from build123d import *

# Parameters (mm, degrees)
SKETCH1_R                = 1.1
SKETCH1_W                = 10
SKETCH1_H                = 2.49
BOSS_EXTRUDE1_DEPTH      = 1.67
SKETCH2_W                = 9.5
SKETCH2_H                = 9.5
BOSS_EXTRUDE2_DEPTH      = 5
SKETCH3_R                = 3.75
BOSS_EXTRUDE3_DEPTH      = 1
FILLET1_R                = 1
SKETCH4_W                = 9.5
SKETCH4_H                = 4.61
BOSS_EXTRUDE4_DEPTH      = 1
SKETCH5_W                = 8.8
SKETCH5_H                = 3.91
BOSS_EXTRUDE5_DEPTH      = 2
CHAMFER1_SIZE            = 0.65
BOSS_EXTRUDE6_DEPTH      = 2.75
BOSS_EXTRUDE6_DEPTH_BACK = 2.75
SKETCH7_W                = 22
SKETCH7_H                = 1
BOSS_EXTRUDE7_DEPTH      = 2.6
SKETCH9_W                = 21.8
SKETCH9_H                = 4
BOSS_EXTRUDE8_DEPTH      = 2.5


with BuildPart() as part:
    # Sketch1 → Boss-Extrude1 (new body)
    with BuildSketch(Plane.XY):
        with BuildLine():
            Line((-10.5, -11.93), (10.5, -11.93))
            ThreePointArc((10.5, -11.93), (11.914213562, -11.344213562), (12.5, -9.93))
            Line((12.5, -9.93), (12.5, 9.93))
            ThreePointArc((12.5, 9.93), (11.914213562, 11.344213562), (10.5, 11.93))
            Line((10.5, 11.93), (-10.5, 11.93))
            ThreePointArc((-10.5, 11.93), (-11.914213562, 11.344213562), (-12.5, 9.93))
            Line((-12.5, 9.93), (-12.5, -9.93))
            ThreePointArc((-12.5, -9.93), (-11.914213562, -11.344213562), (-10.5, -11.93))
        make_face()
        with Locations((-10.5, 9.93)):
            Circle(SKETCH1_R, mode=Mode.SUBTRACT)
        with Locations((10.5, 9.93)):
            Circle(SKETCH1_R, mode=Mode.SUBTRACT)
        with Locations((-10.5, -2.57)):
            Circle(SKETCH1_R, mode=Mode.SUBTRACT)
        with Locations((10.5, -2.57)):
            Circle(SKETCH1_R, mode=Mode.SUBTRACT)
        with Locations((0, 4.965)):
            Rectangle(SKETCH1_W, SKETCH1_H, mode=Mode.SUBTRACT)
    extrude(amount=BOSS_EXTRUDE1_DEPTH)

    # Sketch2 → Boss-Extrude2 (add)
    with BuildSketch(Plane.XY.offset(1.67)):
        with Locations((0, -2.57)):
            Rectangle(SKETCH2_W, SKETCH2_H)
    extrude(amount=BOSS_EXTRUDE2_DEPTH)

    # Sketch3 → Boss-Extrude3 (add)
    with BuildSketch(Plane.XY.offset(6.67)):
        with Locations((0, -2.57)):
            Circle(SKETCH3_R)
    extrude(amount=BOSS_EXTRUDE3_DEPTH)

    # Fillet1
    fillet1_edges = [part.edges().sort_by_distance(p)[0] for p in [
        (-3.75, -2.57, 7.67),
    ]]
    fillet(fillet1_edges, radius=FILLET1_R - 0.0001)  # a hair under: the kernel refuses the full size

    # Sketch4 → Boss-Extrude4 (add)
    with BuildSketch(Plane.XY.offset(1.67)):
        with Locations((0, -9.625)):
            Rectangle(SKETCH4_W, SKETCH4_H)
    extrude(amount=BOSS_EXTRUDE4_DEPTH)

    # Sketch5 → Boss-Extrude5 (add)
    with BuildSketch(Plane.XY.offset(2.67)):
        with Locations((0, -9.625)):
            Rectangle(SKETCH5_W, SKETCH5_H)
    extrude(amount=BOSS_EXTRUDE5_DEPTH)

    # Chamfer1
    chamfer1_edges = [part.edges().sort_by_distance(p)[0] for p in [
        (4.4, -9.625, 4.67),
        (0, -7.67, 4.67),
        (-4.4, -9.625, 4.67),
        (0, -11.58, 4.67),
    ]]
    chamfer(chamfer1_edges, length=CHAMFER1_SIZE)

    # Sketch6 → Boss-Extrude6 (add, two sides: drawn at the far end of the back side and taken through both)
    with BuildSketch(Plane(origin=(0, 0, 0), x_dir=(0, 0, -1), z_dir=(1, 0, 0)).offset(-BOSS_EXTRUDE6_DEPTH_BACK)):
        with BuildLine():
            Line((-3.298312235, 2.18), (-3.534834551, 2.18))
            add(Edge.make_bspline(
                [(-3.534834551, 2.18), (-3.534834551, 4.944931667), (-0.47055609, 4.534187875), (0.730328755, 6.849182289), (0.79246314, 7.291776262), (0.79246314, 7.33)],
                knots=[0, 0, 0, 0, 0.784106591, 0.986086671, 1, 1, 1, 1], degree=3))
            Line((0.79246314, 7.33), (0, 7.33))
            Line((0, 7.33), (0, 11.83))
            Line((0, 11.83), (1.2, 11.83))
            Line((1.2, 11.83), (1.2, 7.33))
            Line((1.2, 7.33), (1.028985456, 7.33))
            add(Edge.make_bspline(
                [(-3.298312235, 2.18), (-3.298312235, 2.369708531), (-3.268931161, 2.774833109), (-3.111748266, 3.367193807), (-2.767956088, 3.909628415), (-2.161529025, 4.362480865), (-1.410396471, 4.725696596), (-0.605704822, 5.099255509), (0.165819225, 5.601384629), (0.682287807, 6.265090703), (0.910091228, 6.771630764), (0.98633259, 7.041505733), (1.014862156, 7.172550739), (1.028985456, 7.28085491), (1.028985456, 7.33)],
                knots=[0, 0, 0, 0, 0.0625, 0.125, 0.25, 0.375, 0.5, 0.625, 0.75, 0.875, 0.9375, 0.96875, 0.984375, 1, 1, 1, 1], degree=3))
        make_face()
    extrude(amount=BOSS_EXTRUDE6_DEPTH + BOSS_EXTRUDE6_DEPTH_BACK)

    # Sketch7 → Boss-Extrude7 (add)
    with BuildSketch(Plane(origin=(0, 0, 0), x_dir=(-1, 0, 0), z_dir=(0, 0, -1))):
        with Locations((0, -11.33)):
            Rectangle(SKETCH7_W, SKETCH7_H)
    extrude(amount=BOSS_EXTRUDE7_DEPTH)

    # Sketch9 → Boss-Extrude8 (add)
    with BuildSketch(Plane(origin=(0, 0, 0), x_dir=(-1, 0, 0), z_dir=(0, 0, -1))):
        with Locations((0, -8.83)):
            Rectangle(SKETCH9_W, SKETCH9_H)
    extrude(amount=BOSS_EXTRUDE8_DEPTH)


solid = part.part
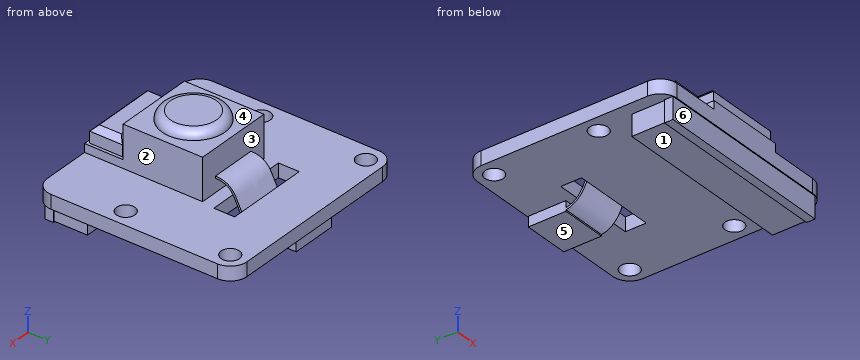
Build history of the part. All positions in model axes, mm. Face numbers are marked on the shaded views. A direction names the side the tool comes from. Coordinates: 2 decimals unless noted, no trailing zeros. Write each loop counter-clockwise with the first axis right and the second up, starting at its lowest first coordinate (ties: lowest second). Pieces come first, ordered by that corner, then holes.
(1) 3-axis set-ups, long thin cutter, end or side, ignore diameter. For the marked faces 4, 5 and 6: which of +Z, -Z, +X, -X, +Y, -Y reach the whole face in a straight line?
(2) Cut at B-B on y = -2.57. State how many separate pieces and enclosed holes the cut face has, and give its area (3 significant figures).
(3) Pin check, flat tips, straight feed: pin 1 Ø1.2 at (y, z) = (-8, -1.5) entering from -X; pin 2 Ø1.5 at (x, z) = (0, 3) entering from +Y; pin 3 Ø1.3 at (x, y) = (-1.5, -9.5) entering from +Z; pin 4 Ø1 at (x, z) = (5.5, 5) entering from +Y. Stop position of each tip, or through.
(4) Cut at A-A on x = 8.75. List the corners of the cut face in (y, z).
(5) Cut at D-D on z = 6.25. List the corners of the cut face in (x, y), and give its area (4 significant figures).
(6) Mould opens along Z. For the marked faces 1, 2 and 3 say: pulls with the +Z half, pulls with the -Z half, needs draft (parallel to the pull), parting line crosses it, or undercut.
(7) Drill centre lines: line 1 (Y direction, x = 10.5, z = 1.05); line 2 (Y direction, x = -1.25, z = 0.5); line 3 (Z direction, x = 1.75, y = 2.25). Where is each one in solid material? Low to high.
(8) Cut at C-C on z = -1.75. List the corners of the cut face in (x, y), and give its area (3 significant figures).
Working result:
1. face 4: +Z
1. face 5: -Z, +X, -X, +Y
1. face 6: -Z, +X, -X, -Y
2. separate pieces: 3
2. enclosed holes: 0
2. area: 89.0 mm2
3. pin 1: stops at x = -10.9
3. pin 2: stops at y = 4.56
3. pin 3: stops at z = 4.67
3. pin 4: passes through
4. outline: (-11.93, 0) - (-11.83, 0) - (-11.83, -2.6) - (-10.83, -2.6) - (-10.83, -2.5) - (-6.83, -2.5) - (-6.83, 0) - (11.93, 0) - (11.93, 1.67) - (-11.93, 1.67) - close
5. outline: (-4.75, -7.32) - (4.75, -7.32) - (4.75, 2.18) - (-4.75, 2.18) - close
5. area: 90.25 mm2
6. face 1: pulls with the -Z half
6. face 2: needs draft
6. face 3: undercut
7. line 1: y = -11.93 to -3.67, -1.47 to 8.83, 11.03 to 11.93
7. line 2: y = -11.93 to 3.72, 5.18 to 5.46, 6.21 to 11.93
7. line 3: z = 0 to 1.67, 3.3 to 3.53
8. outline: (-11, -11.83) - (11, -11.83) - (11, -10.83) - (10.9, -10.83) - (10.9, -6.83) - (-10.9, -6.83) - (-10.9, -10.83) - (-11, -10.83) - close
8. area: 109 mm2
